from build123d import *

# Parameters (mm, degrees)
SKETCH1_W           = 152.4
SKETCH1_H           = 152.4
BOSS_EXTRUDE1_DEPTH = 6.35
SKETCH2_R           = 2.125
CUT_EXTRUDE1_DEPTH  = 6.35
SKETCH3_W           = 6.35
SKETCH3_H           = 6.35
BOSS_EXTRUDE2_DEPTH = 76.2
SKETCH4_W           = 6.35
SKETCH4_H           = 6.384095646
BOSS_EXTRUDE3_DEPTH = 139.7
SKETCH5_W           = 6.35
SKETCH5_H           = 6.384095646
BOSS_EXTRUDE4_DEPTH = 139.7
SKETCH6_W           = 6.35
SKETCH6_H           = 6.384095646
BOSS_EXTRUDE5_DEPTH = 139.7


with BuildPart() as part:
    # Sketch1 → Boss-Extrude1 (new body)
    with BuildSketch(Plane(origin=(0, 0, 0), x_dir=(1, 0, 0), z_dir=(0, 1, 0))):
        with Locations((40.776583963, 45.362139437)):
            Rectangle(SKETCH1_W, SKETCH1_H)
    extrude(amount=BOSS_EXTRUDE1_DEPTH)

    # Sketch2 → Cut-Extrude1 (cut)
    with BuildSketch(Plane(origin=(0, 6.35, 0), x_dir=(1, 0, 0), z_dir=(0, 1, 0))):
        with Locations((0, -2.125)):
            Circle(SKETCH2_R)
        with Locations((0, 55.889)):
            Circle(SKETCH2_R)
    extrude(amount=-CUT_EXTRUDE1_DEPTH, mode=Mode.SUBTRACT)

    # Sketch3 → Boss-Extrude2 (add)
    with BuildSketch(Plane(origin=(0, 6.35, 0), x_dir=(1, 0, 0), z_dir=(0, 1, 0))):
        with Locations((113.801583963, -27.662860563)):
            Rectangle(SKETCH3_W, SKETCH3_H)
        with Locations((-32.248416037, -27.662860563)):
            Rectangle(SKETCH3_W, SKETCH3_H)
        with Locations((-32.248416037, 118.387139437)):
            Rectangle(SKETCH3_W, SKETCH3_H)
        with Locations((113.801583963, 118.387139437)):
            Rectangle(SKETCH3_W, SKETCH3_H)
    extrude(amount=BOSS_EXTRUDE2_DEPTH)

    # Sketch4 → Boss-Extrude3 (add)
    with BuildSketch(Plane(origin=(0, 0, 24.487860563), x_dir=(-1, 0, 0), z_dir=(0, 0, -1))):
        with Locations((-113.801583963, 79.357952177)):
            Rectangle(SKETCH4_W, SKETCH4_H)
        with Locations((32.248416037, 79.357952177)):
            Rectangle(SKETCH4_W, SKETCH4_H)
    extrude(amount=BOSS_EXTRUDE3_DEPTH)

    # Sketch5 → Boss-Extrude4 (add)
    with BuildSketch(Plane(origin=(-29.073416037, 0, 0), x_dir=(0, 0, -1), z_dir=(1, 0, 0))):
        with Locations((-27.662860563, 79.357952177)):
            Rectangle(SKETCH5_W, SKETCH5_H)
        with Locations((118.387139437, 79.357952177)):
            Rectangle(SKETCH5_W, SKETCH5_H)
    extrude(amount=BOSS_EXTRUDE4_DEPTH)

    # Sketch6 → Boss-Extrude5 (add)
    with BuildSketch(Plane(origin=(-29.073416037, 0, 0), x_dir=(0, 0, -1), z_dir=(1, 0, 0))):
        with Locations((45.347085843, 79.357952177)):
            Rectangle(SKETCH6_W, SKETCH6_H)
    extrude(amount=BOSS_EXTRUDE5_DEPTH)


solid = part.part
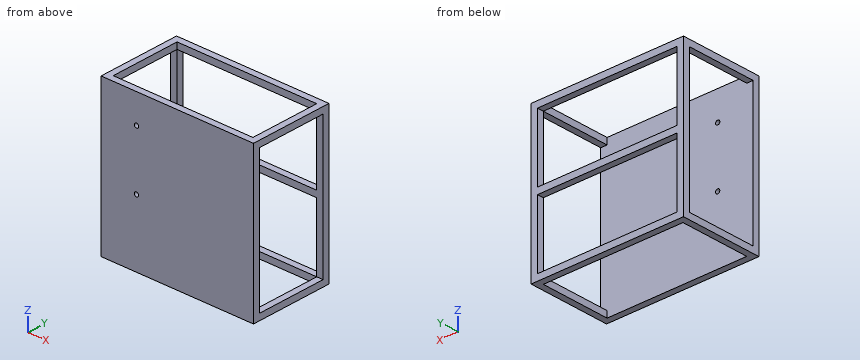
The model under review builds one solid part; all positions refer to its coordinate system, in mm. Round coordinates to 2 decimals unless told otherwise and drop trailing zeros. Loops run counter-clockwise (first coordinate to the right, second up) from the corner with the lowest first, then second, coordinate; pieces in that order, holes last. Notation, with made-up numbers: (9, 38) -> (56, 38) arc R16 ccw to (56, 61) -> close; hole circle Ø10 at (52, -31.75). An arc over 180 degrees is marked (long way). Answer as CSV lines item,"result".
1) For P1, Ø10, axis at y = 10.5, z = 6.5, coming from the +X side; P2, Ø5, axis at x = 100, z = -14, coming from the +Y side, all flat-tipped, find the tip position at first contact; note any pin that passes through.
Geometry results:
P1,"stops at x = 116.98"
P2,"stops at y = 6.35"
2) Add section A-A on x = 0. Write out the cut boundary in (y, z).
Geometry results:
outline,"(0, -121.56) -> (6.35, -121.56) -> (6.35, -58.01) -> (0, -58.01) -> close; (0, -53.76) -> (6.35, -53.76) -> (6.35, 0) -> (0, 0) -> close; (0, 4.25) -> (6.35, 4.25) -> (6.35, 30.84) -> (0, 30.84) -> close; (76.17, -121.56) -> (82.55, -121.56) -> (82.55, -115.21) -> (76.17, -115.21) -> close; (76.17, -48.52) -> (82.55, -48.52) -> (82.55, -42.17) -> (76.17, -42.17) -> close; (76.17, 24.49) -> (82.55, 24.49) -> (82.55, 30.84) -> (76.17, 30.84) -> close"
3) Add section B-B on z = 11. Write out the cut boundary in (x, y), plus the area to 3 significant figures.
Geometry results:
outline,"(-35.42, 0) -> (116.98, 0) -> (116.98, 6.35) -> (-35.42, 6.35) -> close; (-35.42, 76.17) -> (-29.07, 76.17) -> (-29.07, 82.55) -> (-35.42, 82.55) -> close; (110.63, 76.17) -> (116.98, 76.17) -> (116.98, 82.55) -> (110.63, 82.55) -> close"
area,"1,050 mm²"
4) To check wall thickness, follow line 1 along Z through (x, y) = (0, 4); line 2 along Z through (x, y) = (-2.5, 77); line 3 along X through (y, z) = (77, -53). State the ranges of each line that lie inside material, in increasing order. Write a range as from..to.
Geometry results:
line 1,"z = -121.56..-58.01, -53.76..0, 4.25..30.84"
line 2,"z = -121.56..-115.21, -48.52..-42.17, 24.49..30.84"
line 3,"x = -35.42..-29.07, 110.63..116.98"
5) Add section D-D on x = 40.5. Write out the cut boundary in (y, z), plus the area to 3 significant figures.
Geometry results:
outline,"(0, -121.56) -> (6.35, -121.56) -> (6.35, 30.84) -> (0, 30.84) -> close; (76.17, -121.56) -> (82.55, -121.56) -> (82.55, -115.21) -> (76.17, -115.21) -> close; (76.17, -48.52) -> (82.55, -48.52) -> (82.55, -42.17) -> (76.17, -42.17) -> close; (76.17, 24.49) -> (82.55, 24.49) -> (82.55, 30.84) -> (76.17, 30.84) -> close"
area,"1,090 mm²"
6) Add section C-C on y = 32. Write out the cut boundary in (x, z), plus the area to 3 significant figures.
Geometry results:
outline,"(-35.42, -121.56) -> (-29.07, -121.56) -> (-29.07, -115.21) -> (-35.42, -115.21) -> close; (-35.42, 24.49) -> (-29.07, 24.49) -> (-29.07, 30.84) -> (-35.42, 30.84) -> close; (110.63, -121.56) -> (116.98, -121.56) -> (116.98, -115.21) -> (110.63, -115.21) -> close; (110.63, 24.49) -> (116.98, 24.49) -> (116.98, 30.84) -> (110.63, 30.84) -> close"
area,"161 mm²"
